from build123d import *

# Parameters (mm, degrees)
SKETCH_1_W      = 26
SKETCH_1_H      = 72.2
SKETCH_1_R      = 1.1
EXTRUDE_1_DEPTH = 2
SKETCH_2_R      = 1.65
EXTRUDE_2_DEPTH = 2
FILLET_1_R      = 2


with BuildPart() as part:
    # 草图1 → 凸台-拉伸1 (new body)
    with BuildSketch(Plane.XY):
        Rectangle(SKETCH_1_W, SKETCH_1_H)
        with Locations((-10, 24)):
            Circle(SKETCH_1_R, mode=Mode.SUBTRACT)
        with Locations((10, 24)):
            Circle(SKETCH_1_R, mode=Mode.SUBTRACT)
        with Locations((-10, -24)):
            Circle(SKETCH_1_R, mode=Mode.SUBTRACT)
        with Locations((10, -24)):
            Circle(SKETCH_1_R, mode=Mode.SUBTRACT)
    extrude(amount=EXTRUDE_1_DEPTH)

    # 草图2 → 凸台-拉伸2 (add)
    # profile 1 of 2: a face of its own
    with BuildSketch(Plane.XY.offset(2)):
        with BuildLine():
            Line((-8, 42.1), (-8, 36.1))
            Line((-8, 36.1), (0, 36.1))
            Line((0, 36.1), (0, 42.1))
            ThreePointArc((0, 42.1), (-4, 46.1), (-8, 42.1))
        make_face()
        with Locations((-4, 42.1)):
            Circle(SKETCH_2_R, mode=Mode.SUBTRACT)
    # profile 2 of 2: a face of its own
    with BuildSketch(Plane.XY.offset(2)):
        with BuildLine():
            Line((-8, -42.1), (-8, -36.1))
            Line((-8, -36.1), (0, -36.1))
            Line((0, -36.1), (0, -42.1))
            ThreePointArc((0, -42.1), (-4, -46.1), (-8, -42.1))
        make_face()
        with Locations((-4, -42.1)):
            Circle(SKETCH_2_R, mode=Mode.SUBTRACT)
    extrude(amount=-EXTRUDE_2_DEPTH)

    # 圆角1
    fillet_1_edges = [part.edges().sort_by_distance(p)[0] for p in [
        (-8, 36.1, 1),
        (0, 36.1, 1),
        (0, -36.1, 1),
        (-8, -36.1, 1),
        (-13, 36.1, 1),
        (13, 36.1, 1),
        (13, -36.1, 1),
        (-13, -36.1, 1),
    ]]
    fillet(fillet_1_edges, radius=FILLET_1_R)


solid = part.part
Verification items for the finished model (mm, model axes). A direction names the side the tool comes from. Round coordinates to 2 decimals unless told otherwise and drop trailing zeros. Order: outer loops, then holes, each group sorted by start corner. A loop starts at its lowest first (then second) coordinate and runs counter-clockwise, first axis right, second up. Notation, with made-up numbers: (17, 45.25) -> (45, 45.25) arc R22 cw to (45, 71.25) -> close; hole circle Ø11 at (-25, 59). An arc over 180 degrees is marked (long way). Put each result on its own line as item: value.
1) Mould release check, pull along X, two halves, no side actions. Record for faces 1 (the cylindrical face through (-9.492, -24.976, 0.986)), 2 (the flat face through (-8, -40, 1)), 3 (the flat face through (6, 36.1, 1)): +X half, -X half, draft (parallel to the pull), parting line (faces both ways), or undercut.
Final values:
face 1: undercut
face 2: -X half
face 3: draft
2) Material ranges on line 1 (Y direction, x = 10, z = 0.6); line 2 (Y direction, x = -4.25, z = 1.3); line 3 (Y direction, x = 12, z = 0.4), recorded low to high.
Final values:
line 1: y = -36.1 to -25.1, -22.9 to 22.9, 25.1 to 36.1
line 2: y = -46.09 to -43.73, -40.47 to 40.47, 43.73 to 46.09
line 3: y = -35.83 to 35.83
3) Set-up check for faces 4 (the flat face through (0, 40, 1)), 5 (the flat face through (-8, 40, 1)), 6 (the flat face through (6, -36.1, 1)): record each of +Z, -Z, +X, -X, +Y, -Y from which the full face is reachable in a straight line by a thin tool's end or side.
Final values:
face 4: +Z, -Z, +X, +Y
face 5: +Z, -Z, -X, +Y
face 6: +Z, -Z, +X, -Y
4) Depth check by flat-ended pin: pin 1 (0.6 mm diameter, centred on y = 41, z = 1, fed in from +X); pin 2 (0.6 mm diameter, centred on x = 6.5, z = 1, fed in from -Y). Enter the tip coordinate at first touch or a pass-through.
Final values:
pin 1: stops at x = 0
pin 2: stops at y = -36.1
5) Section check A-A (y = 24). Record the cut outline in (x, z).
Final values:
outline: (-13, 0) -> (-11.1, 0) -> (-11.1, 2) -> (-13, 2) -> close; (-8.9, 0) -> (8.9, 0) -> (8.9, 2) -> (-8.9, 2) -> close; (11.1, 0) -> (13, 0) -> (13, 2) -> (11.1, 2) -> close
6) Section check C-C (x = 4.25). Record the cut outline in (y, z).
Final values:
outline: (-36.1, 0) -> (36.1, 0) -> (36.1, 2) -> (-36.1, 2) -> close
7) Section check B-B (z = 1.7). Record the cut outline in (x, y).
Final values:
outline: (-13, -34.1) arc R2 ccw to (-11, -36.1) -> (-10, -36.1) arc R2 cw to (-8, -38.1) -> (-8, -42.1) arc R4 ccw to (0, -42.1) -> (0, -38.1) arc R2 cw to (2, -36.1) -> (11, -36.1) arc R2 ccw to (13, -34.1) -> (13, 34.1) arc R2 ccw to (11, 36.1) -> (2, 36.1) arc R2 cw to (0, 38.1) -> (0, 42.1) arc R4 ccw to (-8, 42.1) -> (-8, 38.1) arc R2 cw to (-10, 36.1) -> (-11, 36.1) arc R2 ccw to (-13, 34.1) -> close; hole circle Ø2.2 at (-10, -24); hole circle Ø2.2 at (-10, 24); hole circle Ø3.3 at (-4, -42.1); hole circle Ø3.3 at (-4, 42.1); hole circle Ø2.2 at (10, -24); hole circle Ø2.2 at (10, 24)
